```python
from build123d import *

# Parameters (mm, degrees)
SKETCH1_R           = 11.6713
BOSS_EXTRUDE1_DEPTH = 23.4442
SKETCH4_R           = 9.3726
BOSS_EXTRUDE3_DEPTH = 3.5814
SKETCH5_R           = 2.9464
BOSS_EXTRUDE4_DEPTH = 0.7366
SKETCH2_R           = 1.0287
BOSS_EXTRUDE2_DEPTH = 10.6426


with BuildPart() as part:
    # Sketch1 → Boss-Extrude1 (new body)
    with BuildSketch(Plane.XY):
        Circle(SKETCH1_R)
    extrude(amount=BOSS_EXTRUDE1_DEPTH)

    # Sketch4 → Boss-Extrude3 (add)
    with BuildSketch(Plane.XY.offset(23.4442)):
        Circle(SKETCH4_R)
    extrude(amount=BOSS_EXTRUDE3_DEPTH)

    # Sketch5 → Boss-Extrude4 (add)
    with BuildSketch(Plane.XY.offset(27.0256)):
        Circle(SKETCH5_R)
    extrude(amount=BOSS_EXTRUDE4_DEPTH)

    # Sketch2 → Boss-Extrude2 (add)
    with BuildSketch(Plane.XY.offset(27.7622)):
        Circle(SKETCH2_R)
    extrude(amount=BOSS_EXTRUDE2_DEPTH)


solid = part.part
```
Could you check a few things on this model? Use its own coordinates, in mm. A direction names the side the tool comes from. Give positions to 0.01 mm unless a question says otherwise; leave off trailing zeros. Loops run counter-clockwise (first coordinate to the right, second up) from the corner with the lowest first, then second, coordinate; pieces in that order, holes last. Notation, with made-up numbers: (53.25, 0.25) - (57.25, 0.25) arc R21 ccw to (57.25, 25.25) - close; hole circle Ø10 at (-13, -39.75). An arc over 180 degrees is marked (long way). Answer in a Markdown table with one row per item. Add a question column.
Q1. If we section it at A-A (x = 0): List the corners of the cut face in (y, z) for me, plus the area to 3 significant figures.
Q2. If we section it at D-D (x = -8.25): List the corners of the cut face in (y, z) for me.
Q3. If we section it at C-C (z = 19): List the corners of the cut face in (x, y) for me, plus the area to 3 significant figures.
Q4. Please list where these lines run through material, in increasing order: L1, parallel to Z at x = -6.75, y = 2.75; L2, parallel to Z at x = 9.25, y = 3.25; L3, parallel to X at y = 0.25, z = 24.5. Write a range as from..to.
Q5. For pin 1 (6 mm diameter, centred on x = -4, z = 23, fed in from +Y); pin 2 (8 mm diameter, centred on x = 8.5, y = -8.5, fed in from +Z); pin 3 (3 mm diameter, centred on x = -9, y = 2.5, fed in from -Z); pin 4 (2 mm diameter, centred on x = -5, z = 6.5, fed in from -Y), each with a flat end and sliding along its axis, tell me the tip position at first contact or that it passes through.
Q6. Which directions (+Z, -Z, +X, -X, +Y, -Y) give clear straight access to the entire face, cutting with the end or side of a thin tool? Please do faces 1 (the face through (0, 0, 0)), 2 (the face through (-1.028, 0.045, 33.009)).
The answers:
| question | item | result |
|---|---|---|
| 1 | outline | (-11.67, 0) - (11.67, 0) - (11.67, 23.44) - (9.37, 23.44) - (9.37, 27.03) - (2.95, 27.03) - (2.95, 27.76) - (1.03, 27.76) - (1.03, 38.4) - (-1.03, 38.4) - (-1.03, 27.76) - (-2.95, 27.76) - (-2.95, 27.03) - (-9.37, 27.03) - (-9.37, 23.44) - (-11.67, 23.44) - close |
| 1 | area | 641 mm^2 |
| 2 | outline | (-8.26, 0) - (8.26, 0) - (8.26, 23.44) - (4.45, 23.44) - (4.45, 27.03) - (-4.45, 27.03) - (-4.45, 23.44) - (-8.26, 23.44) - close |
| 3 | outline | circle Ø23.34 at (0, 0) |
| 3 | area | 428 mm^2 |
| 4 | L1 | z = 0..27.03 |
| 4 | L2 | z = 0..23.44 |
| 4 | L3 | x = -9.37..9.37 |
| 5 | pin 1 | stops at y = 11.63 |
| 5 | pin 2 | stops at z = 27.03 |
| 5 | pin 3 | stops at z = 0 |
| 5 | pin 4 | stops at y = -10.96 |
| 6 | face 1 | -Z, +X, -X, +Y, -Y |
| 6 | face 2 | +Z |
